```python
from build123d import *

# Parameters (mm, degrees)
SKETCH1_W           = 49.53
SKETCH1_H           = 68.58
BOSS_EXTRUDE1_DEPTH = 2.54
SKETCH3_R           = 0.9
BOSS_EXTRUDE3_DEPTH = 12.7
BOSS_EXTRUDE4_START = -5.08
BOSS_EXTRUDE4_DEPTH = 12.7


with BuildPart() as part:
    # Sketch1 → Boss-Extrude1 (new body)
    with BuildSketch(Plane(origin=(0, 0, 0), x_dir=(1, 0, 0), z_dir=(0, 1, 0))):
        Rectangle(SKETCH1_W, SKETCH1_H)
    extrude(amount=BOSS_EXTRUDE1_DEPTH)

    # Sketch3 → Boss-Extrude3 (add)
    with BuildSketch(Plane(origin=(0, 2.54, 0), x_dir=(1, 0, 0), z_dir=(0, 1, 0))):
        with Locations(Location((4.445, -25.4, 0), (0, 0, 90))):
            Circle(SKETCH3_R)
        with Locations(Location((19.685, -25.4, 0), (0, 0, 90))):
            Circle(SKETCH3_R)
    extrude(amount=BOSS_EXTRUDE3_DEPTH)

    # Sketch4 → Boss-Extrude4 (add)
    with BuildSketch(Plane.ZY.offset(24.765).offset(BOSS_EXTRUDE4_START)):
        Polygon((-10.882960378, 2.54), (-10.882960378, 16.234305586), (-8.32780624, 16.234305586), (-8.32780624, 8.89), (10.72219376, 8.89), (10.72219376, 16.234305586), (13.277347899, 16.234305586), (13.277347899, 2.54), align=None)
    extrude(amount=-BOSS_EXTRUDE4_DEPTH)


solid = part.part
```
Work out the finished part from the listing and answer in its coordinate system (mm). A direction names the side the tool comes from. Coordinates: 2 decimals unless noted, no trailing zeros. Loops run counter-clockwise (first coordinate to the right, second up) from the corner with the lowest first, then second, coordinate; pieces in that order, holes last. Notation, with made-up numbers: (85.25, -6) -> (121.25, -6) arc R20 ccw to (121.25, 29) -> close; hole circle Ø10 at (24, 31.5). An arc over 180 degrees is marked (long way). Answer as CSV lines item,"result".
Q1. The part is cut by section C-C on y = 6. Write down the section's boundary in (x, z) (3 decimals), and give its area (3 significant figures).
Findings:
outline,"(-19.685, -10.883) -> (-6.985, -10.883) -> (-6.985, 13.277) -> (-19.685, 13.277) -> close; circle Ø1.8 at (4.445, 25.4); circle Ø1.8 at (19.685, 25.4)"
area,"312 mm²"
Q2. The part is cut by section B-B on z = 25.4. Write down the section's boundary in (x, y) (3 decimals).
Findings:
outline,"(-24.765, 0) -> (24.765, 0) -> (24.765, 2.54) -> (20.585, 2.54) -> (20.585, 15.24) -> (18.785, 15.24) -> (18.785, 2.54) -> (5.345, 2.54) -> (5.345, 15.24) -> (3.545, 15.24) -> (3.545, 2.54) -> (-24.765, 2.54) -> close"
Q3. Find the intervals of material crossed by probe 1 along Z at (x, y) = (-14, 15); probe 2 along Y at (x, z) = (-10.5, -4.5); probe 3 along Y at (x, z) = (16, -16), in increasing order.
Findings:
probe 1,"z = -10.88 to -8.33, 10.72 to 13.28"
probe 2,"y = 0 to 8.89"
probe 3,"y = 0 to 2.54"
Q4. For a pull along Z with two mould halves and no side action, classify faces 1 (the face through (-13, 16.234, -10)), 2 (the face through (20.233, 8.801, 26.114)), 3 (the face through (-13, 13, 10.722)), 4 (the face through (-13, 13, -8.328)) as +Z half, -Z half, draft (parallel to the pull), parting line (faces both ways), or undercut.
Findings:
face 1,"draft"
face 2,"parting line"
face 3,"undercut"
face 4,"undercut"
Q5. A tool of negligible diameter and unlimited length cuts with its end or side. For faces 5 (the face through (-13, 9, 13.277)), 6 (the face through (-13, 9, -10.883)), 7 (the face through (-6.985, 6, 1)), 8 (the face through (4.4, 8.8, 26.3)), 9 (the face through (-19.685, 6, 1)), from which of +Z, -Z, +X, -X, +Y, -Y can it reach the whole face along a straight path? Write none if from no direction.
Findings:
face 5,"+Z, +X, -X, +Y"
face 6,"-Z, +X, -X, +Y"
face 7,"+Z, -Z, +X, +Y"
face 8,"+Y"
face 9,"+Z, -Z, -X, +Y"
Q6. The part is cut by section A-A on y = 11.75. Write down the section's boundary in (x, z) (3 decimals).
Findings:
outline,"(-19.685, -10.883) -> (-6.985, -10.883) -> (-6.985, -8.328) -> (-19.685, -8.328) -> close; (-19.685, 10.722) -> (-6.985, 10.722) -> (-6.985, 13.277) -> (-19.685, 13.277) -> close; circle Ø1.8 at (4.445, 25.4); circle Ø1.8 at (19.685, 25.4)"
Q7. The part is cut by section D-D on x = 2.5. Write down the section's boundary in (y, z), and give its area (3 significant figures).
Findings:
outline,"(0, -34.29) -> (2.54, -34.29) -> (2.54, 34.29) -> (0, 34.29) -> close"
area,"174 mm²"
Q8. Each of these flat-tipped pins is pushed along its axis until it touches: pin 1 (1 mm diameter, centred on x = 18.5, z = -3.5, fed in from -Y); pin 2 (8 mm diameter, centred on x = -11, y = 13, fed in from +Z); pin 3 (1.4 mm diameter, centred on x = 4, z = 25.5, fed in from +Y); pin 4 (6 mm diameter, centred on x = -10, y = 11, fed in from -Z). Where does it stop, or does it pass through?
Findings:
pin 1,"stops at y = 0"
pin 2,"stops at z = 13.28"
pin 3,"stops at y = 15.24"
pin 4,"stops at z = -10.88"
